Read the model definition and answer for the solid it produces. Units are mm, in the model's axes. A direction names the side the tool comes from. Round coordinates to 2 decimals unless told otherwise and drop trailing zeros. Write each loop counter-clockwise with the first axis right and the second up, starting at its lowest first coordinate (ties: lowest second). Pieces come first, ordered by that corner, then holes. Notation, with made-up numbers: (47.5, 42) -> (93.5, 42) arc R18 ccw to (93.5, 56) -> close; hole circle Ø2 at (66, -3). An arc over 180 degrees is marked (long way). Return JSON: item names as keys, results as strings. Group by question number.
(1) For faces 1 (the flat face through (44.45, -144, -396)), 2 (the flat face through (-31.75, -156, -395)), 3 (the cylindrical face through (31.928, -145.146, -394.341)), determine the directions among +Z, -Z, +X, -X, +Y, -Y from which every point of the face is accessible in a straight line to the end or side of a thin tool.
(2) The mould has two halves that part along Y. Classify faces 4 (the flat face through (1, -24, -19.05)), 5 (the cylindrical face through (-38.19, -146.18, -396.13)): released by +Y, released by -Y, zero draft, split by the parting line, or undercut.
(3) A cutting plane is placed at C-C on z = -75.5. Give the vertices of the cut face in (x, y), then the cut area to 3 significant figures.
(4) Straight lines are drawn through the part: line 1 (Y direction, x = 24.5, z = -387.5); line 2 (Y direction, x = -25, z = -103); line 3 (Y direction, x = -33, z = -398). For each, find the intervals that lie inside material, in ascending order.
(5) Given pin 1 (12 mm diameter, centred on x = -19.5, z = -435, fed in from +Y); pin 2 (5 mm diameter, centred on y = -156, z = -392, fed in from +X), each flat-ended and moving along its own axis, determine where each tip first touches the part or whether it passes through.
(6) A cutting plane is placed at D-D on y = -282.5. Give the vertices of the cut face in (x, z).
```python
from build123d import *

# Parameters (mm, degrees)
F1_DEPTH       = 44.45
F1_DEPTH_BACK  = 44.45
F3_D           = 9.525
F3_DEPTH       = 31.75
F3_CBORE_D     = 15.875
F3_CBORE_DEPTH = 25.4
F5_D           = 9.525
F5_CBORE_D     = 15.875
F5_CBORE_DEPTH = 12.7


with BuildPart() as f1:
    # F0 (on Right) → F1 (new body, two sides)
    with BuildSketch(Plane.YZ) as f1_sk:
        Polygon((-253.798136, -744.067323), (-4.154652, -19.05), (-44.45, -19.05), (-289.822394, -731.663176), align=None)
        Polygon((-264.641732, -775.559412), (-253.798136, -744.067323), (-289.822394, -731.663176), (-304.93708, -775.559412), align=None)
    extrude(amount=F1_DEPTH)
    extrude(f1_sk.sketch, amount=-F1_DEPTH_BACK)

    # F3
    with Locations(Plane.YZ.offset(44.45)):
        with Locations((-152.478508, -391.300663)):
            CounterBoreHole(F3_D / 2, F3_CBORE_D / 2, F3_CBORE_DEPTH, depth=F3_DEPTH)

    # F5 (through all)
    with Locations(Plane(origin=(-44.45, 0, 0), x_dir=(0, -1, 0), z_dir=(-1, 0, 0))):
        with Locations((152.478508, -391.300663)):
            CounterBoreHole(F5_D / 2, F5_CBORE_D / 2, F5_CBORE_DEPTH)


solid = f1.part
```
Checks:
{
 "1": {"face 1": "+Z, -Z, +X, +Y, -Y", "face 2": "-X", "face 3": "+X"},
 "2": {"face 4": "zero draft", "face 5": "undercut"},
 "3": {"outline": "(-44.45, -63.89) -> (44.45, -63.89) -> (44.45, -23.59) -> (-44.45, -23.59) -> close", "area": "3,580 mm^2"},
 "4": {"line 1": "y = -171.32 to -159.45, -145.51 to -131.02", "line 2": "y = -73.36 to -33.06", "line 3": "y = -174.93 to -156.74, -148.22 to -134.64"},
 "5": {"pin 1": "stops at y = -145.31", "pin 2": "stops at x = 19.05"},
 "6": {"outline": "(-44.45, -775.56) -> (44.45, -775.56) -> (44.45, -710.4) -> (-44.45, -710.4) -> close"}
}
